Can you work these out from the model? Positions are in its coordinate system, mm. A direction names the side the tool comes from. Round coordinates to 2 decimals unless told otherwise and drop trailing zeros. Loops run counter-clockwise (first coordinate to the right, second up) from the corner with the lowest first, then second, coordinate; pieces in that order, holes last. Notation, with made-up numbers: (-13.75, 67.5) -> (32.25, 67.5) arc R19 cw to (32.25, 78.5) -> close; hole circle Ø11 at (86, -37). An arc over 180 degrees is marked (long way). Write item = value, one per line.
from build123d import *

# Parameters (mm, degrees)
SKETCH1_W                      = 4.5
SKETCH1_H                      = 10
BOSS_EXTRUDE1_DEPTH            = 15.15
BOSS_EXTRUDE1_2_DEPTH          = 15.15
F_1_5MM_DOWEL_HOLE1_AT_2_COUNT = 2
F_1_5MM_DOWEL_HOLE1_AT_2_PITCH = 27.4
SKETCH5_W                      = 31.9
SKETCH5_H                      = 10
SKETCH5_R                      = 2
BOSS_EXTRUDE2_DEPTH            = 12.5
FILLET1_R                      = 3.175
SKETCH6_R                      = 2
CUT_EXTRUDE1_DEPTH             = 15.4
SKETCH7_R                      = 1.575
BOSS_EXTRUDE3_DEPTH            = 2.5
FILLET3_R                      = 1.5
FILLET4_R                      = 1


with BuildPart() as part:
    # Sketch1 → Boss-Extrude1 (new body)
    with BuildSketch(Plane(origin=(0, 0, 0), x_dir=(1, 0, 0), z_dir=(0, 1, 0))):
        with Locations((-13.7, 0)):
            Rectangle(SKETCH1_W, SKETCH1_H)
    extrude(amount=-BOSS_EXTRUDE1_DEPTH)

    # Sketch4 → Ø1.5mm Dowel Hole1 (revolve, cut)
    with BuildSketch(Plane(origin=(-13.7, 0, 0), x_dir=(0, 0, 1), z_dir=(1, 0, 0))):
        Polygon((0, 0), (0, 12), (0.75, 11.549354536), (0.75, 0), align=None)
    f_1_5mm_dowel_hole1 = revolve(axis=Axis((-13.7, 6.35, 0), (0, -1, 0)), mode=Mode.SUBTRACT)



with BuildPart() as body_2:
    # Sketch1 → Boss-Extrude1 2 (new body)
    with BuildSketch(Plane(origin=(0, 0, 0), x_dir=(1, 0, 0), z_dir=(0, 1, 0))):
        with Locations((13.7, 0)):
            Rectangle(SKETCH1_W, SKETCH1_H)
    extrude(amount=-BOSS_EXTRUDE1_2_DEPTH)

    # Ø1.5mm Dowel Hole1 at 2: Ø1.5mm Dowel Hole1 ×2
    with Locations(*[(i * F_1_5MM_DOWEL_HOLE1_AT_2_PITCH, 0, 0) for i in range(1, F_1_5MM_DOWEL_HOLE1_AT_2_COUNT)]):
        add(f_1_5mm_dowel_hole1, mode=Mode.SUBTRACT)


with BuildPart() as part_1:
    add(part.part)

    add(body_2.part)  # Boss-Extrude2 merges body 2
    # Sketch5 → Boss-Extrude2 (add)
    with BuildSketch(Plane.XZ.offset(15.15)):
        Rectangle(SKETCH5_W, SKETCH5_H)
        with Locations(Location((-4.95, 0, 0), (0, 0, 270))):
            Circle(SKETCH5_R, mode=Mode.SUBTRACT)
    extrude(amount=BOSS_EXTRUDE2_DEPTH)

    # Fillet1
    fillet1_edges = [part_1.edges().sort_by_distance(p)[0] for p in [
        (-11.45, -15.15, 0),
        (11.45, -15.15, 0),
    ]]
    fillet(fillet1_edges, radius=FILLET1_R)

    # Sketch6 → Cut-Extrude1 (cut)
    with BuildSketch(Plane.ZY.offset(15.95)):
        with Locations((-1.2, -20.65)):
            Circle(SKETCH6_R)
    extrude(amount=-CUT_EXTRUDE1_DEPTH, mode=Mode.SUBTRACT)

    # Sketch7 → Boss-Extrude3 (add)
    # profile 1 of 2: a face of its own
    with BuildSketch(Plane.XZ.offset(27.65)):
        with BuildLine():
            Line((3.575, 9), (3.575, 5))
            Line((3.575, 5), (-3.575, 5))
            Line((-3.575, 5), (-3.575, 9))
            ThreePointArc((-3.575, 9), (0, 12.575), (3.575, 9))
        make_face()
        with Locations(Location((0, 9, 0), (0, 0, 270))):
            Circle(SKETCH7_R, mode=Mode.SUBTRACT)
    # profile 2 of 2: a face of its own
    with BuildSketch(Plane.XZ.offset(27.65)):
        with BuildLine():
            Line((3.575, -5), (-3.575, -5))
            Line((-3.575, -5), (-3.575, -9))
            ThreePointArc((-3.575, -9), (0, -12.575), (3.575, -9))
            Line((3.575, -9), (3.575, -5))
        make_face()
        with Locations(Location((0, -9, 0), (0, 0, 270))):
            Circle(SKETCH7_R, mode=Mode.SUBTRACT)
    extrude(amount=-BOSS_EXTRUDE3_DEPTH)

    # Fillet3
    fillet3_edges = [part_1.edges().sort_by_distance(p)[0] for p in [
        (3.575, -26.4, 5),
        (-3.575, -26.4, 5),
        (-3.575, -26.4, -5),
        (3.575, -26.4, -5),
    ]]
    fillet(fillet3_edges, radius=FILLET3_R)

    # Fillet4
    fillet4_edges = [part_1.edges().sort_by_distance(p)[0] for p in [
        (0, -25.15, 5),
        (0, -25.15, -5),
    ]]
    fillet(fillet4_edges, radius=FILLET4_R)


solid = part_1.part
1. Suppose I cut it at A-A, the plane y = -7.5. List the corners of the cut face in (x, z) for me.
Entries:
outline = (-15.95, -5) -> (-11.45, -5) -> (-11.45, 5) -> (-15.95, 5) -> close; (11.45, -5) -> (15.95, -5) -> (15.95, 5) -> (11.45, 5) -> close; hole circle Ø1.5 at (-13.7, 0); hole circle Ø1.5 at (13.7, 0)
2. For faces 1 (the flat face through (-2, -25.15, 9)), 2 (the flat face through (-3.575, -26, -8)), 3 (the flat face through (3.575, -26, 8)), 4 (the flat face through (3.575, -26, -8)), 5 (the cylindrical face through (10.5, -14.24, -0.07)), which set-ups out of +Z, -Z, +X, -X, +Y, -Y let a thin tool reach every point of the face, with its end or its side?
Entries:
face_1 = +Z, +X, -X, +Y
face_2 = -Z, -X, +Y, -Y
face_3 = +Z, +X, +Y, -Y
face_4 = -Z, +X, +Y, -Y
face_5 = +Z, -Z, +Y
3. Suppose I cut it at D-D, the plane z = 2.5. List the corners of the cut face in (x, y) for me (3 decimals).
Entries:
outline = (-15.95, -27.65) -> (15.95, -27.65) -> (15.95, 0) -> (11.45, 0) -> (11.45, -11.975) arc R3.175 cw to (8.275, -15.15) -> (-8.275, -15.15) arc R3.175 cw to (-11.45, -11.975) -> (-11.45, 0) -> (-15.95, 0) -> close
4. We'd pull the mould along Z, two halves only. Please class faces 6 (the cylindrical face through (-8.4, -20.6, -3.2)), 7 (the flat face through (11.45, -6, 0)), 8 (the flat face through (0, -17, -5)): released by +Z, released by -Z, zero draft, split by the parting line, or undercut.
Entries:
face_6 = undercut
face_7 = zero draft
face_8 = released by -Z
5. Suppose I cut it at C-C, the plane x = 0. List the corners of the cut face in (y, z) for me (3 decimals).
Entries:
outline = (-27.65, -12.575) -> (-25.15, -12.575) -> (-25.15, -10.575) -> (-27.65, -10.575) -> close; (-27.65, -7.425) -> (-25.15, -7.425) -> (-25.15, -6) arc R1 cw to (-24.15, -5) -> (-15.15, -5) -> (-15.15, 5) -> (-24.15, 5) arc R1 cw to (-25.15, 6) -> (-25.15, 7.425) -> (-27.65, 7.425) -> close; (-27.65, 10.575) -> (-25.15, 10.575) -> (-25.15, 12.575) -> (-27.65, 12.575) -> close
6. Suppose I cut it at B-B, the plane z = -1.2. List the corners of the cut face in (x, y) for me (3 decimals).
Entries:
outline = (-15.95, -27.65) -> (-6.55, -27.65) -> (-6.55, -22.65) -> (-15.95, -22.65) -> close; (-15.95, -18.65) -> (-6.55, -18.65) -> (-6.55, -15.15) -> (-8.275, -15.15) arc R3.175 cw to (-11.45, -11.975) -> (-11.45, 0) -> (-15.95, 0) -> close; (-3.35, -27.65) -> (15.95, -27.65) -> (15.95, 0) -> (11.45, 0) -> (11.45, -11.975) arc R3.175 cw to (8.275, -15.15) -> (-3.35, -15.15) -> (-3.35, -18.65) -> (-0.55, -18.65) -> (-0.55, -22.65) -> (-3.35, -22.65) -> close
7. I'm going to push flat-ended pins straight in: pin 1 (5 mm diameter, centred on x = 9, z = -5, fed in from +Y); pin 2 (0.8 mm diameter, centred on y = -26.5, z = -7.5, fed in from -X) (3 decimals); pin 3 (5 mm diameter, centred on x = -5, z = -8.5, fed in from +Y); pin 4 (10 mm diameter, centred on x = 4.5, y = -14.5, fed in from -Z). Where does each tip first touch, or does it pass through?
Entries:
pin_1 = 0
pin_2 = -3.575
pin_3 = -25.15
pin_4 = -5
8. I need wall thicknesses on line 1 (X direction, y = -6.5, z = 0); line 2 (Z direction, x = 13.7, y = -5.75); line 3 (Y direction, x = -12.25, z = -1.2). Which ranges of each line are inside material? Lowest first, please. Write a range as [from, to].
Entries:
line_1 = [-15.95, -14.45], [-12.95, -11.45], [11.45, 12.95], [14.45, 15.95]
line_2 = [-5, -0.75], [0.75, 5]
line_3 = [-27.65, -22.65], [-18.65, 0]
